Geometry: final body of the model. Coordinates: model frame, mm. A direction names the side the tool comes from. Give positions to 0.01 mm unless a question says otherwise; leave off trailing zeros. Loops run counter-clockwise (first coordinate to the right, second up) from the corner with the lowest first, then second, coordinate; pieces in that order, holes last.
1. Draft query along X for faces 3 (the face through (-2, 7, -4)), 4 (the face through (-118.294, 0.493, -236.434)). Return one class per face: +X half, -X half, draft (parallel to the pull), parting line (faces both ways), or undercut.
2. Access query for faces 1 (the face through (34, 6, -89)), 2 (the face through (126, 0, -94)). Directions: +Z, -Z, +X, -X, +Y, -Y. A direction counts if a zero-diameter tool reaches every point of the face in a straight line with its end or side. Return the directions, or none.
3. Section A-A, the plane z = 46.5. Output: boundary loops of the cut face in (x, y), then the cut area to 3 significant figures.
4. Section B-B, the plane x = 16. Output: boundary loops of the cut face in (y, z).
5. Material intervals for line 1 along X through (y, z) = (4, 247.75); line 2 along X through (y, z) = (1.25, -114); line 3 along Z through (x, y) = (1, 3.25), sorted ascending.
6. First-contact query: P1, Ø8, axis at x = -40.5, z = -197, coming from the -Y side; P2, Ø4, axis at x = -128, z = 0, coming from the +Y side. Flat tips, straight axial feed; report the tip coordinate or a pass-through.
from build123d import *

# Parameters (mm, degrees)
SKETCH1_W                      = 264
SKETCH1_H                      = 500
BOSS_EXTRUDE1_DEPTH            = 7
CUT_EXTRUDE1_DEPTH             = 1
F_3_0MM_DOWEL_HOLE1_AT_2_COUNT = 2
F_3_0MM_DOWEL_HOLE1_AT_2_PITCH = 55
F_3_0MM_DOWEL_HOLE1_AT_3_COUNT = 2
F_3_0MM_DOWEL_HOLE1_AT_3_PITCH = 110
F_3_0MM_DOWEL_HOLE1_AT_4_COUNT = 2
F_3_0MM_DOWEL_HOLE1_AT_4_PITCH = 165
F_3_0MM_DOWEL_HOLE1_AT_5_COUNT = 2
F_3_0MM_DOWEL_HOLE1_AT_5_PITCH = 220
CUT_EXTRUDE2_DEPTH             = 6
FILLET1_R                      = 4
M3_TAPPED_HOLE2_D              = 2.5
M3_TAPPED_HOLE2_DEPTH          = 7.5
M3_TAPPED_HOLE2_TIP            = 0.751075774


with BuildPart() as part:
    # Sketch1 → Boss-Extrude1 (new body)
    with BuildSketch(Plane(origin=(0, 0, 0), x_dir=(1, 0, 0), z_dir=(0, 1, 0))):
        Rectangle(SKETCH1_W, SKETCH1_H)
    extrude(amount=BOSS_EXTRUDE1_DEPTH)

    # Sketch2 → Cut-Extrude1 (cut)
    with BuildSketch(Plane.XZ):
        with BuildLine():
            Line((123, 230), (123, -230))
            ThreePointArc((123, -230), (119.778174593, -237.778174593), (112, -241))
            Line((112, -241), (-112, -241))
            ThreePointArc((-112, -241), (-119.778174593, -237.778174593), (-123, -230))
            Line((-123, -230), (-123, 230))
            ThreePointArc((-123, 230), (-119.778174593, 237.778174593), (-112, 241))
            Line((-112, 241), (112, 241))
            ThreePointArc((112, 241), (119.778174593, 237.778174593), (123, 230))
        make_face()
        with BuildLine():
            Line((121, 230), (121, -230))
            ThreePointArc((121, -230), (118.363961031, -236.363961031), (112, -239))
            Line((112, -239), (-112, -239))
            ThreePointArc((-112, -239), (-118.363961031, -236.363961031), (-121, -230))
            Line((-121, -230), (-121, 230))
            ThreePointArc((-121, 230), (-118.363961031, 236.363961031), (-112, 239))
            Line((-112, 239), (112, 239))
            ThreePointArc((112, 239), (118.363961031, 236.363961031), (121, 230))
        make_face(mode=Mode.SUBTRACT)
    extrude(amount=-CUT_EXTRUDE1_DEPTH, mode=Mode.SUBTRACT)

    # Sketch3 → Ø3.0mm Dowel Hole1 (revolve, cut)
    with BuildSketch(Plane(origin=(128, 7, 220), x_dir=(0, 0, 1), z_dir=(1, 0, 0))):
        Polygon((0, 0), (0, 15.901290929), (1.5, 15), (1.5, 0), align=None)
    f_3_0mm_dowel_hole1 = revolve(axis=Axis((128, 13.35, 220), (0, -1, 0)), mode=Mode.SUBTRACT)

    # Ø3.0mm Dowel Hole1 at 2: Ø3.0mm Dowel Hole1 ×2
    with Locations(*[(0, 0, -i * F_3_0MM_DOWEL_HOLE1_AT_2_PITCH) for i in range(1, F_3_0MM_DOWEL_HOLE1_AT_2_COUNT)]):
        add(f_3_0mm_dowel_hole1, mode=Mode.SUBTRACT)

    # Ø3.0mm Dowel Hole1 at 3: Ø3.0mm Dowel Hole1 ×2
    with Locations(*[(0, 0, -i * F_3_0MM_DOWEL_HOLE1_AT_3_PITCH) for i in range(1, F_3_0MM_DOWEL_HOLE1_AT_3_COUNT)]):
        add(f_3_0mm_dowel_hole1, mode=Mode.SUBTRACT)

    # Ø3.0mm Dowel Hole1 at 4: Ø3.0mm Dowel Hole1 ×2
    with Locations(*[(0, 0, -i * F_3_0MM_DOWEL_HOLE1_AT_4_PITCH) for i in range(1, F_3_0MM_DOWEL_HOLE1_AT_4_COUNT)]):
        add(f_3_0mm_dowel_hole1, mode=Mode.SUBTRACT)

    # Ø3.0mm Dowel Hole1 at 5: Ø3.0mm Dowel Hole1 ×2
    with Locations(*[(0, 0, -i * F_3_0MM_DOWEL_HOLE1_AT_5_PITCH) for i in range(1, F_3_0MM_DOWEL_HOLE1_AT_5_COUNT)]):
        add(f_3_0mm_dowel_hole1, mode=Mode.SUBTRACT)

    # Mirror1: Ø3.0mm Dowel Hole1 across plane
    add(f_3_0mm_dowel_hole1.mirror(Plane.XY), mode=Mode.SUBTRACT)

    # Mirror1 copy 1 sketch → Mirror1 copy 1 (revolve, cut)
    with BuildSketch(Plane(origin=(128, 7, -165), x_dir=(0, 0, -1), z_dir=(1, 0, 0))):
        Polygon((0, 0), (0, -15.901290929), (1.5, -15), (1.5, 0), align=None)
    revolve(axis=Axis((128, 13.35, -165), (0, 1, 0)), mode=Mode.SUBTRACT)

    # Mirror1 copy 2 sketch → Mirror1 copy 2 (revolve, cut)
    with BuildSketch(Plane(origin=(128, 7, -110), x_dir=(0, 0, -1), z_dir=(1, 0, 0))):
        Polygon((0, 0), (0, -15.901290929), (1.5, -15), (1.5, 0), align=None)
    revolve(axis=Axis((128, 13.35, -110), (0, 1, 0)), mode=Mode.SUBTRACT)

    # Mirror1 copy 3 sketch → Mirror1 copy 3 (revolve, cut)
    with BuildSketch(Plane(origin=(128, 7, -55), x_dir=(0, 0, -1), z_dir=(1, 0, 0))):
        Polygon((0, 0), (0, -15.901290929), (1.5, -15), (1.5, 0), align=None)
    revolve(axis=Axis((128, 13.35, -55), (0, 1, 0)), mode=Mode.SUBTRACT)

    # Mirror1 copy 4 sketch → Mirror1 copy 4 (revolve, cut)
    with BuildSketch(Plane(origin=(128, 7, 0), x_dir=(0, 0, -1), z_dir=(1, 0, 0))):
        Polygon((0, 0), (0, -15.901290929), (1.5, -15), (1.5, 0), align=None)
    revolve(axis=Axis((128, 13.35, 0), (0, 1, 0)), mode=Mode.SUBTRACT)

    # Mirror2: Ø3.0mm Dowel Hole1 across plane
    add(f_3_0mm_dowel_hole1.mirror(Plane(origin=(0, 0, 0), x_dir=(0, 0, 1), z_dir=(1, 0, 0))), mode=Mode.SUBTRACT)

    # Mirror2 copy 1 sketch → Mirror2 copy 1 (revolve, cut)
    with BuildSketch(Plane(origin=(-128, 7, -220), x_dir=(0, 0, -1), z_dir=(-1, 0, 0))):
        Polygon((0, 0), (0, 15.901290929), (1.5, 15), (1.5, 0), align=None)
    revolve(axis=Axis((-128, 13.35, -220), (0, -1, 0)), mode=Mode.SUBTRACT)

    # Mirror2 copy 2 sketch → Mirror2 copy 2 (revolve, cut)
    with BuildSketch(Plane(origin=(-128, 7, -165), x_dir=(0, 0, -1), z_dir=(-1, 0, 0))):
        Polygon((0, 0), (0, 15.901290929), (1.5, 15), (1.5, 0), align=None)
    revolve(axis=Axis((-128, 13.35, -165), (0, -1, 0)), mode=Mode.SUBTRACT)

    # Mirror2 copy 3 sketch → Mirror2 copy 3 (revolve, cut)
    with BuildSketch(Plane(origin=(-128, 7, -110), x_dir=(0, 0, -1), z_dir=(-1, 0, 0))):
        Polygon((0, 0), (0, 15.901290929), (1.5, 15), (1.5, 0), align=None)
    revolve(axis=Axis((-128, 13.35, -110), (0, -1, 0)), mode=Mode.SUBTRACT)

    # Mirror2 copy 4 sketch → Mirror2 copy 4 (revolve, cut)
    with BuildSketch(Plane(origin=(-128, 7, -55), x_dir=(0, 0, -1), z_dir=(-1, 0, 0))):
        Polygon((0, 0), (0, 15.901290929), (1.5, 15), (1.5, 0), align=None)
    revolve(axis=Axis((-128, 13.35, -55), (0, -1, 0)), mode=Mode.SUBTRACT)

    # Mirror2 copy 5 sketch → Mirror2 copy 5 (revolve, cut)
    with BuildSketch(Plane(origin=(-128, 7, 0), x_dir=(0, 0, -1), z_dir=(-1, 0, 0))):
        Polygon((0, 0), (0, 15.901290929), (1.5, 15), (1.5, 0), align=None)
    revolve(axis=Axis((-128, 13.35, 0), (0, -1, 0)), mode=Mode.SUBTRACT)

    # Mirror2 copy 6 sketch → Mirror2 copy 6 (revolve, cut)
    with BuildSketch(Plane(origin=(-128, 7, 165), x_dir=(0, 0, 1), z_dir=(-1, 0, 0))):
        Polygon((0, 0), (0, -15.901290929), (1.5, -15), (1.5, 0), align=None)
    revolve(axis=Axis((-128, 13.35, 165), (0, 1, 0)), mode=Mode.SUBTRACT)

    # Mirror2 copy 7 sketch → Mirror2 copy 7 (revolve, cut)
    with BuildSketch(Plane(origin=(-128, 7, 110), x_dir=(0, 0, 1), z_dir=(-1, 0, 0))):
        Polygon((0, 0), (0, -15.901290929), (1.5, -15), (1.5, 0), align=None)
    revolve(axis=Axis((-128, 13.35, 110), (0, 1, 0)), mode=Mode.SUBTRACT)

    # Mirror2 copy 8 sketch → Mirror2 copy 8 (revolve, cut)
    with BuildSketch(Plane(origin=(-128, 7, 55), x_dir=(0, 0, 1), z_dir=(-1, 0, 0))):
        Polygon((0, 0), (0, -15.901290929), (1.5, -15), (1.5, 0), align=None)
    revolve(axis=Axis((-128, 13.35, 55), (0, 1, 0)), mode=Mode.SUBTRACT)

    # Mirror2 copy 9 sketch → Mirror2 copy 9 (revolve, cut)
    with BuildSketch(Plane(origin=(-128, 7, 0), x_dir=(0, 0, 1), z_dir=(-1, 0, 0))):
        Polygon((0, 0), (0, -15.901290929), (1.5, -15), (1.5, 0), align=None)
    revolve(axis=Axis((-128, 13.35, 0), (0, 1, 0)), mode=Mode.SUBTRACT)

    # Sketch5 → Cut-Extrude2 (cut)
    with BuildSketch(Plane(origin=(0, 0, 0), x_dir=(-1, 0, 0), z_dir=(0, -1, 0))):
        Polygon((112, -230), (-112, -230), (112, -10), align=None)
        Polygon((97.728720398, -10), (-112, -215.983564676), (-112, -10), align=None)
        Polygon((-112, 10), (97.728720398, 10), (-112, 215.983564676), align=None)
        Polygon((112, 10), (112, 230), (-112, 230), align=None)
    extrude(amount=-CUT_EXTRUDE2_DEPTH, mode=Mode.SUBTRACT)

    # Fillet1
    fillet1_edges = [part.edges().sort_by_distance(p)[0] for p in [
        (-112, 3, 10),
        (-112, 3, 230),
        (112, 3, 230),
        (112, 3, 10),
        (-97.728720398, 3, 10),
        (112, 3, 215.983564676),
        (112, 3, -10),
        (112, 3, -215.983564676),
        (-97.728720398, 3, -10),
        (-112, 3, -10),
        (112, 3, -230),
        (-112, 3, -230),
    ]]
    fillet(fillet1_edges, radius=FILLET1_R)

    # M3 Tapped Hole2
    with Locations(Plane.XY.offset(250)):
        with Locations((-129, 4), (-39, 4), (39, 4), (129, 4)):
            Hole(M3_TAPPED_HOLE2_D / 2, depth=M3_TAPPED_HOLE2_DEPTH)
            with Locations((0, 0, -(M3_TAPPED_HOLE2_DEPTH + M3_TAPPED_HOLE2_TIP / 2))):  # 118° drill point
                Cone(0, M3_TAPPED_HOLE2_D / 2, M3_TAPPED_HOLE2_TIP, mode=Mode.SUBTRACT)


solid = part.part
Answers below:
1. face 3: draft
1. face 4: undercut
2. face 1: -Y
2. face 2: +Z, -Z, +X, -X, -Y
3. outline: (-132, 0) - (-123, 0) - (-123, 1) - (-121, 1) - (-121, 0) - (-112, 0) - (-112, 6) - (-74.84, 6) - (-74.84, 0) - (-60.57, 0) - (-60.57, 6) - (112, 6) - (112, 0) - (121, 0) - (121, 1) - (123, 1) - (123, 0) - (132, 0) - (132, 7) - (-132, 7) - close
3. area: 586 mm2
4. outline: (0, -250) - (7, -250) - (7, 250) - (0, 250) - (0, 241) - (1, 241) - (1, 239) - (0, 239) - (0, 230) - (6, 230) - (6, 135.71) - (0, 135.71) - (0, 121.7) - (6, 121.7) - (6, 10) - (0, 10) - (0, -10) - (6, -10) - (6, -121.7) - (0, -121.7) - (0, -135.71) - (6, -135.71) - (6, -230) - (0, -230) - (0, -239) - (1, -239) - (1, -241) - (0, -241) - close
5. line 1: x = -132 to -130.25, -127.75 to -40.25, -37.75 to 37.75, 40.25 to 127.75, 130.25 to 132
5. line 2: x = -132 to -112, -6.11 to 8.16, 112 to 132
5. line 3: z = -250 to -230, -120.98 to -106.97, -10 to 10, 106.97 to 120.98, 230 to 250
6. P1: stops at y = 6
6. P2: stops at y = 7
